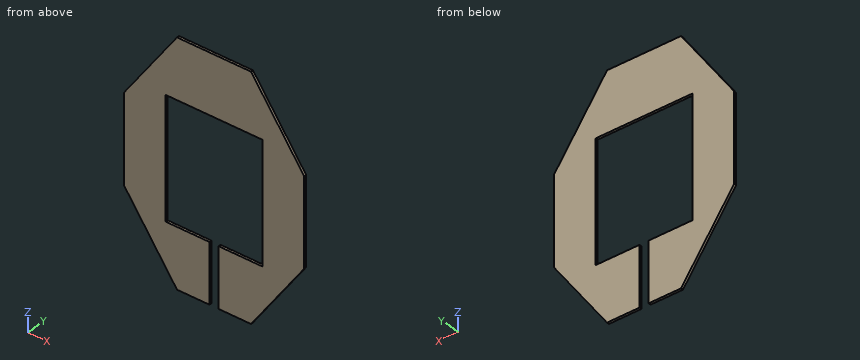
from build123d import *

# Parameters (mm, degrees)
SKETCH1_W           = 33
SKETCH1_H           = 43
BOSS_EXTRUDE1_DEPTH = 0.65
CUT_EXTRUDE1_DEPTH  = 0.25
SKETCH3_W           = 16
SKETCH3_H           = 20
CUT_EXTRUDE2_DEPTH  = 4.125
CUT_EXTRUDE3_DEPTH  = 4.125
SKETCH5_W           = 1.5
SKETCH5_H           = 10
CUT_EXTRUDE4_DEPTH  = 10
SKETCH6_W           = 7.307736582
SKETCH6_H           = 22.967172114
SKETCH6_W_2         = 20.795730386
SKETCH6_H_2         = 8.393457445
SKETCH6_W_3         = 19.542864514
SKETCH6_H_3         = 6.295941965
SKETCH6_W_4         = 6.096070792
CUT_EXTRUDE5_DEPTH  = 5


with BuildPart() as part:
    # Sketch1 → Boss-Extrude1 (new body)
    with BuildSketch(Plane(origin=(0, 0, 0), x_dir=(1, 0, 0), z_dir=(0, 1, 0))):
        Rectangle(SKETCH1_W, SKETCH1_H)
    extrude(amount=BOSS_EXTRUDE1_DEPTH)

    # Sketch2 → Cut-Extrude1 (cut)
    with BuildSketch(Plane.XZ):
        Polygon((5, 21.5), (16.5, 21.5), (16.5, 5), (15, 5), (15, -5), (16.5, -5), (16.5, -21.5), (5, -21.5), (5, -20), (-5, -20), (-5, -21.5), (-16.5, -21.5), (-16.5, -5), (-15, -5), (-15, 5), (-16.5, 5), (-16.5, 21.5), (-5, 21.5), (-5, 20), (5, 20), align=None)
    extrude(amount=-CUT_EXTRUDE1_DEPTH, mode=Mode.SUBTRACT)

    # Sketch3 → Cut-Extrude2 (cut)
    with BuildSketch(Plane.XZ.offset(-0.25)):
        Rectangle(SKETCH3_W, SKETCH3_H)
    extrude(amount=-CUT_EXTRUDE2_DEPTH, mode=Mode.SUBTRACT)

    # Sketch4 → Cut-Extrude3 (cut)
    with BuildSketch(Plane.XZ.offset(-0.25)):
        Polygon((-5, 21.5), (-16.5, 5), (-16.5, 21.5), align=None)
        Polygon((5, 21.5), (16.5, 5), (16.5, 21.5), align=None)
        Polygon((-16.5, -5), (-5, -21.5), (-16.5, -21.5), align=None)
        Polygon((16.5, -5), (5, -21.5), (16.5, -21.5), align=None)
    extrude(amount=-CUT_EXTRUDE3_DEPTH, mode=Mode.SUBTRACT)

    # Sketch5 → Cut-Extrude4 (cut)
    with BuildSketch(Plane.XZ.offset(-0.25)):
        with Locations((0, -15)):
            Rectangle(SKETCH5_W, SKETCH5_H)
    extrude(amount=-CUT_EXTRUDE4_DEPTH, mode=Mode.SUBTRACT)

    # Sketch6 → Cut-Extrude5 (cut, symmetric)
    with BuildSketch(Plane.XZ.offset(-0.25)):
        with Locations((18.553868291, 0.304489024)):
            Rectangle(SKETCH6_W, SKETCH6_H)
        with Locations((0.125275484, 24.096728723)):
            Rectangle(SKETCH6_W_2, SKETCH6_H_2)
        with Locations((-0.501157452, -23.047970983)):
            Rectangle(SKETCH6_W_3, SKETCH6_H_3)
        with Locations((-17.948035396, 0.304489024)):
            Rectangle(SKETCH6_W_4, SKETCH6_H)
    extrude(amount=CUT_EXTRUDE5_DEPTH, both=True, mode=Mode.SUBTRACT)


solid = part.part
Can you work these out from the model? Positions are in its coordinate system, mm. Round coordinates to 2 decimals unless told otherwise and drop trailing zeros. Write each loop counter-clockwise with the first axis right and the second up, starting at its lowest first coordinate (ties: lowest second). Pieces come first, ordered by that corner, then holes. Notation, with made-up numbers: (73.5, 10) - (80.5, 10) arc R19 ccw to (80.5, 19) - close; hole circle Ø1 at (-17.75, -24.75). An arc over 180 degrees is marked (long way). Write each question's results on one line, items separated by ' | '. Start each with the question number.
1) Suppose I cut it at B-B (x = 1.75). List the corners of the cut face in (y, z) for me.
2) Suppose I cut it at C-C (y = 0.45). List the corners of the cut face in (x, z) for me.
3) Suppose I cut it at D-D (x = -12.5). List the corners of the cut face in (y, z) for me.
4) Please list where these lines run through material, in increasing order: line 1 (Z direction, x = -3, y = 0.55); line 2 (Z direction, x = -6.5, y = 0.3); line 3 (X direction, y = 0.5, z = -14).
5) Suppose I cut it at A-A (z = -5.5). List the corners of the cut face in (x, y) for me, and give its area (3 significant figures).
Here are the results:
1) outline: (0.25, -19.9) - (0.65, -19.9) - (0.65, -10) - (0.25, -10) - close; (0.25, 10) - (0.65, 10) - (0.65, 19.9) - (0.25, 19.9) - close
2) outline: (-14.9, -7.3) - (-6.12, -19.9) - (-0.75, -19.9) - (-0.75, -10) - (-8, -10) - (-8, 10) - (8, 10) - (8, -10) - (0.75, -10) - (0.75, -19.9) - (6.12, -19.9) - (14.9, -7.3) - (14.9, 7.3) - (6.12, 19.9) - (-6.12, 19.9) - (-14.9, 7.3) - close
3) outline: (0.25, -10.74) - (0.65, -10.74) - (0.65, 10.74) - (0.25, 10.74) - close
4) line 1: z = -19.9 to -10, 10 to 19.9 | line 2: z = -19.35 to -10, 10 to 19.35 | line 3: x = -10.23 to -0.75, 0.75 to 10.23
5) outline: (-14.9, 0.25) - (-8, 0.25) - (-8, 0.65) - (-14.9, 0.65) - close; (8, 0.25) - (14.9, 0.25) - (14.9, 0.65) - (8, 0.65) - close | area: 5.52 mm2
